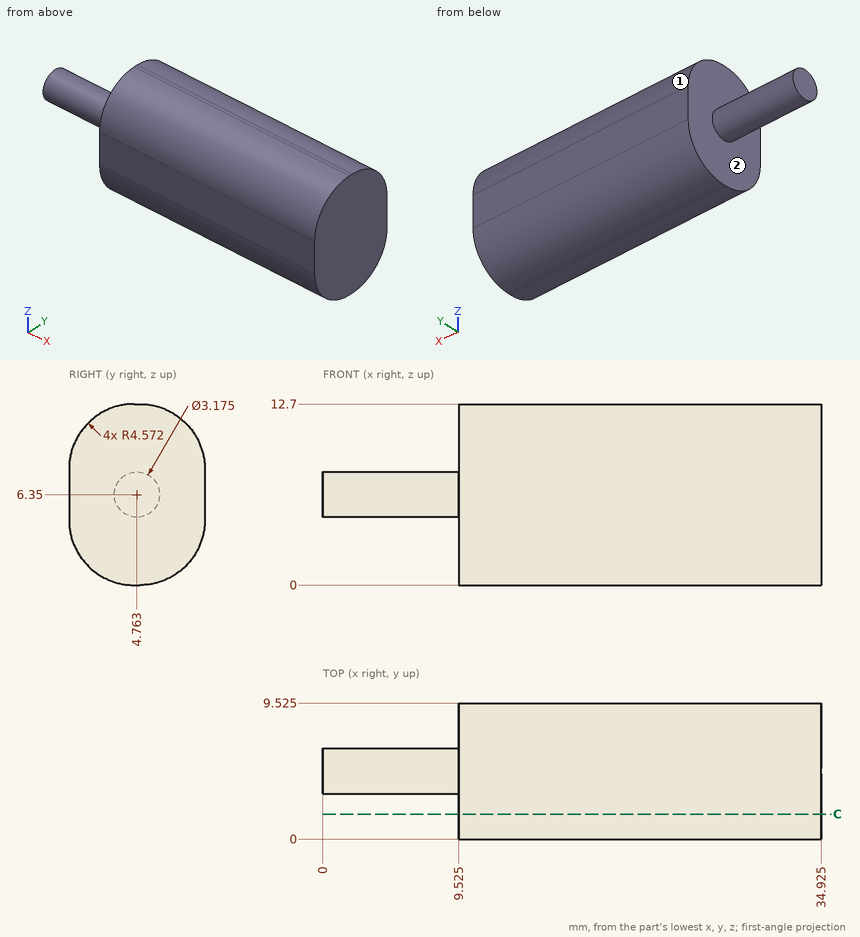
Verification items for this drawing (mm, ordinates from the low corner). A direction names the side the tool comes from. Give positions to 0.01 mm unless a question says otherwise; leave off trailing zeros. Write each loop counter-clockwise with the first axis right and the second up, starting at its lowest first coordinate (ties: lowest second). Pieces come first, ordered by that corner, then holes.
1) Cross-section at C-C (y = 1.75). Record the boundary of the cut face in (x, z) (1 decimal), plus the area to 3 significant figures.
Values follow:
outline: (9.5, 1) - (34.9, 1) - (34.9, 11.7) - (9.5, 11.7) - close
area: 273 mm2
2) Set-up check for the marked faces 1 and 2: record each of +Z, -Z, +X, -X, +Y, -Y from which the full face is reachable in a straight line by a thin tool's end or side.
Values follow:
face 1: +Z, +X, -X, +Y
face 2: -X
3) Go/stop test with flat-tipped pins: pin 1 Ø4 at (x, y) = (28, 8) entering from -Z; pin 2 Ø3 at (y, z) = (3.5, 6.5) entering from -X; pin 3 Ø6 at (x, z) = (4, 7) entering from -Y (1 decimal); pin 4 Ø6 at (x, z) = (4, 10.5) entering from -Y. Record where each tip stops, or that it passes through.
Values follow:
pin 1: stops at z = 0.12
pin 2: stops at x = 0
pin 3: stops at y = 3.2
pin 4: stops at y = 3.67
4) Thickness scan on line 1 (X direction, y = 6.25, z = 1) (1 decimal); line 2 (Z direction, x = 27, y = 2.75); line 3 (Z direction, x = 14, y = 6.25). Record the ranges inside material, lowest first.
Values follow:
line 1: x = 9.5 to 34.9
line 2: z = 0.38 to 12.32
line 3: z = 0.19 to 12.51
